Build history of the part. All positions in model axes, mm. A direction names the side the tool comes from. Give positions to 0.01 mm unless a question says otherwise; leave off trailing zeros. Loops run counter-clockwise (first coordinate to the right, second up) from the corner with the lowest first, then second, coordinate; pieces in that order, holes last. Notation, with made-up numbers: (88, 41) -> (126, 41) arc R27 ccw to (126, 64) -> close; hole circle Ø9 at (76, -36). An arc over 180 degrees is marked (long way). One line per question, with ' | ' between items. Start each with the question number.
(1) Flat gauge pin, fed straight in: pin 1 Ø5 at (y, z) = (-32, 22.5) entering from +X. Where does the tip first touch, or does it go through?
(2) Slice it at B-B, the plane y = -25. Write the cut outline in (x, z), then the cut area to 3 significant figures.
(3) 3-axis set-ups, long thin cutter, end or side, ignore diameter. For faces 1 (the face through (46.896, -9.951, 0.986)), 2 (the face through (6, -2, 8)), 3 (the face through (10, 0, 10)): which of +Z, -Z, +X, -X, +Y, -Y reach the whole face in a straight line?
(4) Slice it at D-D, the plane z = 31. Write the cut outline in (x, y), then the cut area to 3 significant figures.
(5) Drill centre lines: L1, parallel to Y at x = 1, z = 46; L2, parallel to Y at x = 8, z = 9; L3, parallel to Z at x = 0.5, y = -9.5. Where is each one in solid material? Low to high. Write a range as from..to.
(6) Slice it at A-A, the plane z = 46.5. Write the cut outline in (x, y).
(7) Slice it at C-C, the plane x = 22.5. Write the cut outline in (y, z).
(8) Mould opens along Z. For faces 4 (the face through (1, -2, 50)), 5 (the face through (0.99, -9.12, 44.79)), 6 (the face through (52, -25, 1)) say: pulls with the +Z half, pulls with the -Z half, needs draft (parallel to the pull), parting line crosses it, or undercut.
```python
from build123d import *

# Parameters (mm, degrees)
F1_DEPTH = 50
F3_DEPTH = 2
F5_DEPTH = 2
F7_DEPTH = 52.001
F8_R     = 11
F8_R_2   = 1.75
F9_DEPTH = 52.001
F10_SIZE = 4


with BuildPart() as f1:
    # F0 (on Front) → F1 (new body)
    with BuildSketch(Plane.XZ):
        with BuildLine():
            Line((2, 52), (0, 52))
            Line((0, 52), (0, 2.292893))
            ThreePointArc((0, 2.292893), (0.671573, 0.671573), (2.292893, 0))
            Line((2.292893, 0), (52, 0))
            Line((52, 0), (52, 2))
            Line((52, 2), (3, 2))
            ThreePointArc((3, 2), (2.292893, 2.292893), (2, 3))
            Line((2, 3), (2, 52))
        make_face()
    extrude(amount=F1_DEPTH)

    # F2 (on face) → F3 (join)
    with BuildSketch(Plane.XZ.offset(50)):
        Polygon((17, 2), (2, 22), (2, 2), align=None)
    extrude(amount=-F3_DEPTH)

    # F4 (on face) → F5 (join)
    with BuildSketch(Plane(origin=(0, 0, 0), x_dir=(-1, 0, 0), z_dir=(0, 1, 0))):
        Polygon((-2, 2), (-2, 22), (-17, 2), align=None)
    extrude(amount=-F5_DEPTH)

    # F6 (on face) → F7 (cut, through all)
    with BuildSketch(Plane(origin=(0, 0, 0), x_dir=(1, 0, 0), z_dir=(0, 0, -1))):
        with BuildLine():
            Line((27.146447, 37.75), (44.646447, 37.75))
            ThreePointArc((44.646447, 37.75), (46.896447, 40), (44.646447, 42.25))
            Line((44.646447, 42.25), (27.146447, 42.25))
            Line((27.146447, 42.25), (9.646447, 42.25))
            ThreePointArc((9.646447, 42.25), (7.396447, 40), (9.646447, 37.75))
            Line((9.646447, 37.75), (27.146447, 37.75))
        make_face()
        with BuildLine():
            Line((27.146447, 12.25), (9.646447, 12.25))
            ThreePointArc((9.646447, 12.25), (7.396447, 10), (9.646447, 7.75))
            Line((9.646447, 7.75), (27.146447, 7.75))
            Line((27.146447, 7.75), (44.646447, 7.75))
            ThreePointArc((44.646447, 7.75), (46.896447, 10), (44.646447, 12.25))
            Line((44.646447, 12.25), (27.146447, 12.25))
        make_face()
    extrude(amount=-F7_DEPTH, mode=Mode.SUBTRACT)

    # F8 (on face) → F9 (cut, through all)
    with BuildSketch(Plane(origin=(0, 0, 0), x_dir=(0, -1, 0), z_dir=(-1, 0, 0))):
        with Locations((25, 31)):
            Circle(F8_R)
        with Locations((9.5, 46.5)):
            Circle(F8_R_2)
        with Locations((9.5, 15.5)):
            Circle(F8_R_2)
        with Locations((40.5, 15.5)):
            Circle(F8_R_2)
        with Locations((40.5, 46.5)):
            Circle(F8_R_2)
    extrude(amount=-F9_DEPTH, mode=Mode.SUBTRACT)

    # F10
    f10_edges = [f1.edges().sort_by_distance(p)[0] for p in [
        (1, 0, 52),
        (1, -50, 52),
        (52, 0, 1),
        (52, -50, 1),
    ]]
    chamfer(f10_edges, length=F10_SIZE)


solid = f1.part
```
Final values:
1) pin 1: x = 2
2) outline: (0, 2.29) arc R2.29 ccw to (2.29, 0) -> (52, 0) -> (52, 2) -> (3, 2) arc R1 cw to (2, 3) -> (2, 20) -> (0, 20) -> close; (0, 42) -> (2, 42) -> (2, 52) -> (0, 52) -> close | area: 159 mm2
3) face 1: +Z, -Z | face 2: +Z, +X | face 3: +Z, -Z, +X, -X, +Y
4) outline: (0, -50) -> (2, -50) -> (2, -36) -> (0, -36) -> close; (0, -14) -> (2, -14) -> (2, 0) -> (0, 0) -> close | area: 56.0 mm2
5) L1: -50..-42.18, -38.82..-11.18, -7.82..0 | L2: -50..-48, -2..0 | L3: 0.86..13.75, 17.25..44.75, 48.25..52
6) outline: (0, -50) -> (2, -50) -> (2, -42.25) -> (0, -42.25) -> close; (0, -38.75) -> (2, -38.75) -> (2, -11.25) -> (0, -11.25) -> close; (0, -7.75) -> (2, -7.75) -> (2, 0) -> (0, 0) -> close
7) outline: (-50, 0) -> (-42.25, 0) -> (-42.25, 2) -> (-50, 2) -> close; (-37.75, 0) -> (-12.25, 0) -> (-12.25, 2) -> (-37.75, 2) -> close; (-7.75, 0) -> (0, 0) -> (0, 2) -> (-7.75, 2) -> close
8) face 4: pulls with the +Z half | face 5: undercut | face 6: needs draft
